Can you work these out from the model? Positions are in its coordinate system, mm. A direction names the side the tool comes from. Coordinates: 2 decimals unless noted, no trailing zeros. Answer as CSV lines item,"result". Start each with the question number.
1. If we mould it in two halves opening along Y, with no side actions, what happens to faces 1 (the face through (17.92, 197.52, 1.97)), 2 (the face through (-37.832, -22.473, 1.972)), 3 (the face through (-33.86, 14.49, 1.97)), 4 (the face through (-1, 88, 0))? For each: released by +Y, released by -Y, zero draft, split by the parting line, or undercut.
2. I need wall thicknesses on line 1 along Y through (x, z) = (-13.5, 1.25); line 2 along Y through (x, z) = (-18.25, 1.1); line 3 along Y through (x, z) = (-19.5, 3.7). Which ranges of each line are inside material? Lowest first, please. Write a range as from..to.
3. If we section it at A-A (z = 2.1): Give the number of separate pieces and of enclosed holes in the cut face, plus the area to 3 significant figures.
4. On a 3-axis mill with a long thin cutter (end or side, diameter ignored), from which of +Z, -Z, +X, -X, +Y, -Y can I reach the whole of each face in a straight line? I mean faces 5 (the face through (-0.242, 73.577, 1.972)), 6 (the face through (-0.757, 237.492, 1.972)). Say none if no direction works.
5. Will these pins go through, and if not, where does the flat tip stop? pin 1 (1.5 mm diameter, centred on y = 36, z = 1, fed in from -X); pin 2 (1.5 mm diameter, centred on y = -10, z = 2.5, fed in from +X); pin 3 (2 mm diameter, centred on y = 45.5, z = 1.5, fed in from +X).
Autodesk Inventor part; units mm, degrees
ref_plane "YZ Plane" through (0, 0, 0) normal (1, 0, 0) x (0, 1, 0)
ref_plane "XZ Plane" through (0, 0, 0) normal (0, 1, 0) x (-1, 0, 0)
ref_plane "XY Plane" through (0, 0, 0) normal (0, 0, 1) x (1, 0, 0)
sketch "Sketch1" plane through (0, 0, 0) normal (0, 0, 1) x (1, 0, 0)
  line L0 (0, 0) -> (0, 200) construction
  arc A0 (37.1934, 204.7857) -> (-37.1934, 204.7857) centre (0, 200) ccw
  line L1 (0, 200) -> (-18.25, 200) construction
  circle A1 centre (-18.25, 200) radius 2.5
  line L2 (0, 200) -> (18.25, 200) construction
  circle A2 centre (18.25, 200) radius 2.5
  circle A3 centre (0, 0) radius 15
  line L3 (37.1934, 204.7857) -> (59.7122, 29.7756)
  line L4 (-37.1934, 204.7857) -> (-59.9286, 28.0941)
  line L5 (48.4528, 117.2807) -> (43.4937, 116.6426) construction
  line L6 (51.1509, 57.1332) -> (35.8365, 176.152) construction
  circle A4 centre (35.8365, 176.152) radius 1.5
  circle A5 centre (51.1509, 57.1332) radius 1.5
  circle A6 centre (43.4937, 116.6426) radius 1.5
  line L7 (0, 237.5) -> (0, 232.5) construction
  circle A7 centre (0, 232.5) radius 1.5
  circle A8 centre (-35.8365, 176.152) radius 1.5
  circle A9 centre (-51.1509, 57.1332) radius 1.5
  circle A10 centre (-43.4937, 116.6426) radius 1.5
  circle A11 centre (0, 200) radius 4.75
  line L8 (0, 200) -> (0, 60.58) construction
  circle A12 centre (0, 60.58) radius 11 construction
  line L9 (0, 62.58) -> (0, 58.58) construction
  arc A13 (-11, 58.58) -> (11, 58.58) centre (0, 58.58) ccw
  line L10 (-11, 62.58) -> (-11, 58.58)
  line L11 (11, 62.58) -> (11, 58.58)
  arc A14 (11, 62.58) -> (-11, 62.58) centre (0, 62.58) ccw
  line L12 (-15.5, 60.58) -> (15.5, 60.58) construction
  line L13 (0, 76.08) -> (0, 45.08) construction
  circle A15 centre (-15.5, 45.08) radius 1.5 construction
  line L14 (-15.5, 47.08) -> (-15.5, 43.08) construction
  arc A16 (-14, 47.08) -> (-16.9989, 47.0217) centre (-15.5, 47.08) ccw
  line L15 (-14, 47.08) -> (-14, 43.08)
  line L16 (-17, 43.08) -> (-17, 47.08)
  arc A17 (-17, 43.08) -> (-14, 43.08) centre (-15.5, 43.08) ccw
  circle A18 centre (15.5, 45.08) radius 1.5 construction
  line L17 (15.5, 47.08) -> (15.5, 43.08) construction
  arc A19 (16.9989, 47.0217) -> (14, 47.08) centre (15.5, 47.08) ccw
  line L18 (14, 47.08) -> (14, 43.08)
  line L19 (17, 43.08) -> (17, 47.08)
  arc A20 (14, 43.08) -> (17, 43.08) centre (15.5, 43.08) ccw
  circle A21 centre (-15.5, 76.08) radius 1.5 construction
  line L20 (-15.5, 74.08) -> (-15.5, 78.08) construction
  arc A22 (-16.9989, 74.1383) -> (-14, 74.08) centre (-15.5, 74.08) ccw
  line L21 (-14, 74.08) -> (-14, 78.08)
  line L22 (-17, 78.08) -> (-17, 74.08)
  arc A23 (-14, 78.08) -> (-17, 78.08) centre (-15.5, 78.08) ccw
  arc A24 (17, 78.08) -> (14, 78.08) centre (15.5, 78.08) ccw
  circle A25 centre (15.5, 76.08) radius 1.5 construction
  line L23 (14, 74.08) -> (14, 78.08)
  line L24 (15.5, 74.08) -> (15.5, 78.08) construction
  line L25 (17, 78.08) -> (17, 74.08)
  arc A26 (14, 74.08) -> (16.9989, 74.1383) centre (15.5, 74.08) ccw
  circle A27 centre (0, 0) radius 45 construction
  circle A28 centre (0, -45) radius 9.5
  circle A29 centre (0, -45) radius 14.5 construction
  circle A30 centre (0, -59.5) radius 2.25
  circle A31 centre (14.5, -45) radius 2.25
  circle A32 centre (0, -30.5) radius 2.25
  circle A33 centre (-14.5, -45) radius 2.25
  circle A34 centre (0, -45) radius 21.5 construction
  circle A35 centre (38.9711, 22.5) radius 21.5 construction
  circle A36 centre (51.5285, 29.75) radius 2.25 construction
  circle A37 centre (46.2211, 9.9426) radius 2.25 construction
  circle A38 centre (31.7211, 35.0574) radius 2.25 construction
  circle A39 centre (26.4138, 15.25) radius 2.25 construction
  circle A40 centre (38.9711, 22.5) radius 9.5
  circle A41 centre (-38.9711, 22.5) radius 21.5 construction
  circle A42 centre (-51.5285, 29.75) radius 2.25 construction
  circle A43 centre (-31.7211, 35.0574) radius 2.25 construction
  circle A44 centre (-46.2211, 9.9426) radius 2.25 construction
  circle A45 centre (-26.4138, 15.25) radius 2.25 construction
  circle A46 centre (-38.9711, 22.5) radius 9.5
  line L26 (-18.6195, -55.75) -> (-57.5907, 11.75)
  line L27 (18.6195, -55.75) -> (57.5907, 11.75)
  line L28 (48.4528, 117.2807) -> (48.4528, 23.0901) construction
  line L29 (59.7122, 29.7756) -> (60.2953, 25.2438)
  line L30 (48.4528, 23.0901) -> (48.4528, -26.9099) construction
  line L31 (48.4528, -26.9099) -> (38.566, -21.2018) construction
  line L32 (38.566, -21.2018) -> (34.2359, -18.7018) construction
  circle A47 centre (34.2359, -18.7018) radius 1.5
  circle A48 centre (-34.2359, -18.7018) radius 1.5
  arc A49 (57.5907, 11.75) -> (60.2953, 25.2438) centre (38.9711, 22.5) ccw
  arc A50 (-60.2953, 25.2438) -> (-57.5907, 11.75) centre (-38.9711, 22.5) ccw
  arc A51 (-18.6195, -55.75) -> (18.6195, -55.75) centre (0, -45) ccw
  circle A52 centre (38.9711, 22.5) radius 14.5 construction
  circle A53 centre (53.4711, 22.5) radius 2.25
  line L33 (38.9711, 22.5) -> (53.4711, 22.5) construction
  circle A54 centre (38.9711, 37) radius 2.25
  circle A55 centre (24.4711, 22.5) radius 2.25
  circle A56 centre (38.9711, 8) radius 2.25
  circle A57 centre (-53.4711, 22.5) radius 2.25
  circle A58 centre (-38.9711, 37) radius 2.25
  circle A59 centre (-24.4711, 22.5) radius 2.25
  circle A60 centre (-38.9711, 8) radius 2.25
  line L34 (-59.9286, 28.0941) -> (-60.2953, 25.2438)
  dimension "d79" = 90
  dimension "d81" = 29
  dimension "d99" = 29
  dimension "L_Elo" = 200
  dimension "D_Junta2" = 75
  dimension "d13" = 18.25
  dimension "d14" = 5
  dimension "D_furoZ" = 30
  dimension "d16" = 5
  dimension "d17" = 120
  dimension "d18" = 3
  dimension "d19" = 3
  dimension "d20" = 3
  dimension "d21" = 5
  dimension "d22" = 3
  dimension "D_Eixo" = 9.5
  dimension "CA" = 139.42
  dimension "DN" = 22
  dimension "NN" = 4
  dimension "d51" = 22
  dimension "d53" = 11
  dimension "d54" = 31
  dimension "d55" = 31
  dimension "FN" = 3
  dimension "d57" = 15.5
  dimension "d58" = 15.5
  dimension "d59" = 4
  dimension "d61" = 3
  dimension "d62" = 1.5
  dimension "d80" = 19
  dimension "d82" = 4.5
  dimension "d83" = 45
  dimension "d84" = 14.5
  dimension "d85" = 14.5
  dimension "d88" = 360
  dimension "d90" = 43
  dimension "d93" = 360
  dimension "d95" = 94.1906
  dimension "d96" = 50
  dimension "d97" = 5
  dimension "d98" = 3
  dimension "d100" = 4.5
  dimension "d104" = 360
extrude "Extrusion1" add sketch "Sketch1" along normal blind 4
equation "\"d16\" = LF"
equation "\"d18\" = D_Sup"
equation "\"d19\" = D_Sup"
equation "\"d20\" = D_Sup"
equation "\"d21\" = LF"
equation "\"d22\" = D_Sup"
properties part number "1ELO"
Solved:
1,face 1,"undercut"
1,face 2,"released by -Y"
1,face 3,"undercut"
1,face 4,"zero draft"
2,line 1,"-61.73..-47.02, -42.98..-6.54, 6.54..234.99"
2,line 2,"-56.37..197.5, 202.5..232.76"
2,line 3,"-54.22..197.83, 202.17..232.03"
3,separate pieces,"1"
3,enclosed holes,"33"
3,area,"23,900 mm²"
4,face 5,"+Z, -Z"
4,face 6,"+Z, -Z, +Y"
5,pin 1,"x = -59.01"
5,pin 2,"x = 45.47"
5,pin 3,"x = 57.82"
